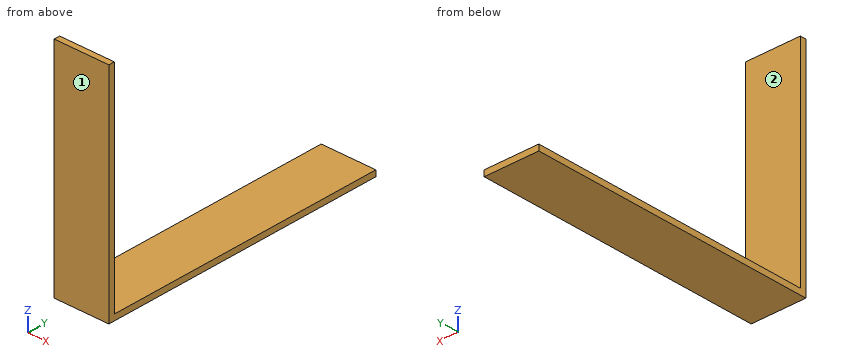
Autodesk Inventor part; units mm, degrees
ref_plane "YZ Plane" through (0, 0, 0) normal (1, 0, 0) x (0, 1, 0)
ref_plane "XZ Plane" through (0, 0, 0) normal (0, 1, 0) x (-1, 0, 0)
ref_plane "XY Plane" through (0, 0, 0) normal (0, 0, 1) x (1, 0, 0)
sketch "Sketch1" plane through (0, 0, 0) normal (1, 0, 0) x (0, 1, 0)
  line L0 (0, 0) -> (134, 0)
  line L1 (134, 0) -> (134, -2.75)
  line L2 (134, -2.75) -> (0, -2.75)
  line L3 (0, -2.75) -> (0, 0)
  line L4 (0, 0) -> (2.75, 0)
  line L5 (2.75, 0) -> (2.75, 100)
  line L6 (2.75, 100) -> (0, 100)
  line L7 (0, 100) -> (0, 0)
  dimension "d0" = 134
  dimension "d1" = 2.75
  dimension "d2" = 2.75
  dimension "d3" = 100
extrude "Extrusion1" add sketch "Sketch1" against normal blind 25.4
properties part number "PLETINA NEMA CAJA"
Here's how the part is built. I have some questions about the finished solid (model axes, mm). Face numbers are marked on the shaded views. A direction names the side the tool comes from. Round coordinates to 2 decimals unless told otherwise and drop trailing zeros. Write each loop counter-clockwise with the first axis right and the second up, starting at its lowest first coordinate (ties: lowest second). Pieces come first, ordered by that corner, then holes. Notation, with made-up numbers: M 34,71 L 79,71 A28 ccw 79,100 Z; hole C 32,-6.5 d9. An arc over 180 degrees is marked long. Answer as CSV lines item,"result". Start each with the question number.
1. Suppose I cut it at C-C on y = 113.5. Write out the boundary of the cut face in (x, z), then the cut area to 4 significant figures.
2. I'm going to push flat-ended pins straight in: pin 1 Ø12.5 at (x, z) = (-18, 56.5) entering from +Y; pin 2 Ø12.5 at (x, y) = (-15, 75) entering from +Z; pin 3 Ø8 at (x, z) = (-11.5, 34.5) entering from -Y. Where does each tip first touch, or does it pass through?
3. I need wall thicknesses on probe 1 along Y at (x, z) = (-10.25, 7); probe 2 along Z at (x, y) = (-13, 84). Which ranges of each line are inside material? Lowest first, please.
4. Suppose I cut it at B-B on z = 71.5. Write out the boundary of the cut face in (x, y), then the cut area to 4 significant figures.
5. Suppose I cut it at A-A on x = -6.75. Write out the boundary of the cut face in (y, z), then the cut area to 4 significant figures.
6. On a 3-axis mill with a long thin cutter (end or side, diameter ignored), from which of +Z, -Z, +X, -X, +Y, -Y can I reach the whole of each face in a straight line? I mean the marked faces 1 and 2. Say none if no direction works.
Check result:
1,outline,"M -25.4,-2.75 L 0,-2.75 L 0,0 L -25.4,0 Z"
1,area,"69.85 mm2"
2,pin 1,"stops at y = 2.75"
2,pin 2,"stops at z = 0"
2,pin 3,"stops at y = 0"
3,probe 1,"y = 0 to 2.75"
3,probe 2,"z = -2.75 to 0"
4,outline,"M -25.4,0 L 0,0 L 0,2.75 L -25.4,2.75 Z"
4,area,"69.85 mm2"
5,outline,"M 0,-2.75 L 134,-2.75 L 134,0 L 2.75,0 L 2.75,100 L 0,100 Z"
5,area,"643.5 mm2"
6,face 1,"+Z, -Z, +X, -X, -Y"
6,face 2,"+Z, +X, -X, +Y"
